from build123d import *

# Parameters (mm, degrees)
RESSALTO_EXTRUS_O1_DEPTH          = 38.1
CORTE_EXTRUS_O1_START             = -10
CORTE_EXTRUS_O1_DEPTH             = 4.5
FURO_COM_FOLGA_DE_M41_D           = 4.5
FURO_COM_FOLGA_DE_M41_DEPTH       = 10
FURO_COM_FOLGA_DE_M41_CSINK_D     = 4.55
FURO_COM_FOLGA_DE_M41_CSINK_ANGLE = 90


with BuildPart() as part:
    # Esboço1 → Ressalto-extrusão1 (new body, symmetric)
    with BuildSketch(Plane.XY):
        Polygon((-4.5, -7.794228634), (4.5, -7.794228634), (9, 0), (4.5, 7.794228634), (-4.5, 7.794228634), (-9, 0), align=None)
    extrude(amount=RESSALTO_EXTRUS_O1_DEPTH, both=True)

    # Esboço4 → Corte-extrusão1 (cut)
    with BuildSketch(Plane.XY.offset(38.1).offset(CORTE_EXTRUS_O1_START)):
        Polygon((2.165063509, 3.75), (-6.834936491, 3.75), (-9, 0), (-6.834936491, -3.75), (2.165063509, -3.75), (4.330127019, 0), align=None)
    corte_extrus_o1 = extrude(amount=-CORTE_EXTRUS_O1_DEPTH, mode=Mode.SUBTRACT)

    # Furo com folga de M41
    with Locations(Plane.XY.offset(38.1)):
        with Locations((0, 0)):
            furo_com_folga_de_m41 = CounterSinkHole(FURO_COM_FOLGA_DE_M41_D / 2, FURO_COM_FOLGA_DE_M41_CSINK_D / 2, depth=FURO_COM_FOLGA_DE_M41_DEPTH, counter_sink_angle=FURO_COM_FOLGA_DE_M41_CSINK_ANGLE)

    # Espelhar1: Corte-extrusão1, Furo com folga de M41 across plane
    add(corte_extrus_o1.mirror(Plane.XY), mode=Mode.SUBTRACT)
    add(furo_com_folga_de_m41.mirror(Plane.XY), mode=Mode.SUBTRACT)


solid = part.part
CAD build for the part. Positions are in the model's coordinates, mm. A direction names the side the tool comes from. Give positions to 0.01 mm unless a question says otherwise; leave off trailing zeros. Order: outer loops, then holes, each group sorted by start corner. A loop starts at its lowest first (then second) coordinate and runs counter-clockwise, first axis right, second up. Notation, with made-up numbers: (85, 0) -> (123, 0) arc R18 cw to (123, 35) -> close; hole circle Ø2 at (7, 21.5). An arc over 180 degrees is marked (long way). Return JSON: item names as keys, results as strings.
Q1. Saw through at B-B (x = 0). Write the cut outline in (y, z) (3 decimals).
Working result:
{"outline": "(-7.794, -38.1) -> (-2.275, -38.1) -> (-2.25, -38.075) -> (-2.25, -28.1) -> (-3.75, -28.1) -> (-3.75, -23.6) -> (3.75, -23.6) -> (3.75, -28.1) -> (2.25, -28.1) -> (2.25, -38.075) -> (2.275, -38.1) -> (7.794, -38.1) -> (7.794, 38.1) -> (2.275, 38.1) -> (2.25, 38.075) -> (2.25, 28.1) -> (3.75, 28.1) -> (3.75, 23.6) -> (-3.75, 23.6) -> (-3.75, 28.1) -> (-2.25, 28.1) -> (-2.25, 38.075) -> (-2.275, 38.1) -> (-7.794, 38.1) -> close"}
Q2. Flat gauge pins, fed straight in: pin 1 (3.5 mm diameter, centred on x = 0, y = 0, fed in from -Z); pin 2 (3 mm diameter, centred on x = 5, z = -25.5, fed in from -Y); pin 3 (4 mm diameter, centred on y = -5, z = -13.5, fed in from +X); pin 4 (2 mm diameter, centred on y = -3, z = -6, fed in from -X). Where does each tip first touch, or does it go through?
Working result:
{"pin 1": "z = -23.6", "pin 2": "y = -7.79", "pin 3": "x = 7.27", "pin 4": "x = -7.85"}
Q3. Saw through at D-D (y = 5.5). Write the cut outline in (x, z), then the cut area to 3 significant figures.
Working result:
{"outline": "(-5.82, -38.1) -> (5.82, -38.1) -> (5.82, 38.1) -> (-5.82, 38.1) -> close", "area": "888 mm²"}
Q4. Drill centre lines: line 1 (Z direction, x = -2.25, y = -0.75); line 2 (X direction, y = 0, z = -34.5); line 3 (Y direction, x = 0, z = -34). Where is each one in solid material? Low to high.
Working result:
{"line 1": "-38.1 to -28.1, -23.6 to 23.6, 28.1 to 38.1", "line 2": "-9 to -2.25, 2.25 to 9", "line 3": "-7.79 to -2.25, 2.25 to 7.79"}
Q5. Which spindle directions (+Z, -Z, +X, -X, +Y, -Y) get a long thin tool onto all of the face, cutting with end or side? Do faces 1 (the face through (0.29, 2.23, -33.02)), 2 (the face through (-2, -3.75, -26)), 3 (the face through (0.29, 2.23, 33.02)). Say none if no direction does.
Working result:
{"face 1": "-Z", "face 2": "-X", "face 3": "+Z"}
Q6. Mould opens along Z. For faces 4 (the face through (3.26, 1.85, 25.88)), 5 (the face through (0, 7.794, 1)), 6 (the face through (2, 2, -38.1)) say: pulls with the +Z half, pulls with the -Z half, needs draft (parallel to the pull), parting line crosses it, or undercut.
Working result:
{"face 4": "undercut", "face 5": "needs draft", "face 6": "pulls with the -Z half"}
Q7. Saw through at C-C (x = -5.25). Write the cut outline in (y, z).
Working result:
{"outline": "(-6.5, -38.1) -> (6.5, -38.1) -> (6.5, 38.1) -> (-6.5, 38.1) -> close; hole (-3.75, -28.1) -> (3.75, -28.1) -> (3.75, -23.6) -> (-3.75, -23.6) -> close; hole (-3.75, 23.6) -> (3.75, 23.6) -> (3.75, 28.1) -> (-3.75, 28.1) -> close"}
Q8. Saw through at A-A (z = 26.5). Write the cut outline in (x, y), then the cut area to 3 significant figures.
Working result:
{"outline": "(-6.83, -3.75) -> (-4.5, -7.79) -> (4.5, -7.79) -> (9, 0) -> (4.5, 7.79) -> (-4.5, 7.79) -> (-6.83, 3.75) -> (2.17, 3.75) -> (4.33, 0) -> (2.17, -3.75) -> close", "area": "127 mm²"}
